```python
from build123d import *

# Parameters (mm, degrees)
F0_W     = 50.8
F0_H     = 38.1
F0_R     = 6.35
F1_DEPTH = 12.446
F2_W     = 1.417765
F2_H     = 38.1
F3_DEPTH = 2.54
F5_DEPTH = 38.1
F6_R     = 2.931554
F7_DEPTH = 12.7


with BuildPart() as f1:
    # F0 (on Top) → F1 (new body)
    with BuildSketch(Plane.XY):
        Rectangle(F0_W, F0_H)
        Circle(F0_R, mode=Mode.SUBTRACT)
    extrude(amount=F1_DEPTH)

    # F2 (on face) → F3 (cut)
    with BuildSketch(Plane.XY.offset(12.446)):
        with Locations((-17.610003, 0)):
            Rectangle(F2_W, F2_H)
        with BuildLine():
            Line((3.892783, 19.05), (0, 19.05))
            Line((0, 19.05), (0, 6.35))
            ThreePointArc((0, 6.35), (2.057368, 6.007473), (3.892783, 5.016846))
            Line((3.892783, 5.016846), (3.892783, 19.05))
        make_face()
        with BuildLine():
            Line((0, -6.35), (0, -19.05))
            Line((0, -19.05), (3.892783, -19.05))
            Line((3.892783, -19.05), (3.892783, -5.016846))
            ThreePointArc((3.892783, -5.016846), (2.057368, -6.007473), (0, -6.35))
        make_face()
    extrude(amount=-F3_DEPTH, mode=Mode.SUBTRACT)

    # F4 (on face) → F5 (cut)
    with BuildSketch(Plane.XZ.offset(19.05)):
        Polygon((14.809987, 12.446), (10.999987, 12.446), (8.067048, 7.366), (14.809987, 7.366), align=None)
        Polygon((18.619987, 12.446), (14.809987, 12.446), (14.809987, 7.366), (21.552927, 7.366), align=None)
    extrude(amount=-F5_DEPTH, mode=Mode.SUBTRACT)

    # F6 (on face) → F7 (join)
    with BuildSketch(Plane.YZ.offset(25.4)):
        with Locations((0, 6.223)):
            Circle(F6_R)
    extrude(amount=F7_DEPTH)


solid = f1.part
```
Geometry check sheet. Reference: the model listing, model coordinates, mm. A direction names the side the tool comes from. Round coordinates to 2 decimals unless told otherwise and drop trailing zeros. Order: outer loops, then holes, each group sorted by start corner. A loop starts at its lowest first (then second) coordinate and runs counter-clockwise, first axis right, second up. Notation, with made-up numbers: (9, 80.5) -> (58, 80.5) arc R33 ccw to (58, 118.5) -> close; hole circle Ø9 at (41.5, 8.5). An arc over 180 degrees is marked (long way). Return JSON: item names as keys, results as strings. Group by question number.
Q1. Section check D-D, the plane z = 5.5. Record the boundary of the cut face in (x, y), plus the area to 3 significant figures.
Q2. Section check C-C, the plane y = -7. Record the boundary of the cut face in (x, z), plus the area to 3 significant figures.
Q3. Section check A-A, the plane y = 0. Record the boundary of the cut face in (x, z), plus the area to 3 significant figures.
Q4. Tool access check on faces 1 (the flat face through (0, -13, 11)), 2 (the flat face through (15, 0, 7.366)), 3 (the flat face through (0, -19.05, 6)), 4 (the cylindrical face through (31.661, -0.636, 3.361)), 5 (the cylindrical face through (-6.344, 0.279, 6.136)). Record the directions out of +Z, -Z, +X, -X, +Y, -Y that give a thin tool (end or side, any length) a straight path to the whole face; none if there is none.
Q5. Gauge pin test, flat ends, axial feed: pin 1 (0.8 mm diameter, centred on y = 10, z = 11.5, fed in from +X); pin 2 (1.1 mm diameter, centred on x = -17.5, y = 1.5, fed in from +Z). Record the tip position at first contact, or that the pin passes through.
Q6. Release check for a two-part mould opening along X. For faces 6 (the flat face through (-18.319, 0, 11)), 7 (the flat face through (5, 5, 0)), 8 (the flat face through (25.4, 0, 2)) record: released by +X, released by -X, zero draft, split by the parting line, or undercut.
Q7. Section check B-B, the plane z = 11.5. Record the boundary of the cut face in (x, y).
Q8. Material ranges on probe 1 along Y at (x, z) = (0, 2.75); probe 2 along X at (y, z) = (0, 3.5); probe 3 along X at (y, z) = (10.5, 12.25), recorded low to high. Write a range as from..to.
Numbers:
{
 "1": {"outline": "(-25.4, -19.05) -> (25.4, -19.05) -> (25.4, -2.84) -> (38.1, -2.84) -> (38.1, 2.84) -> (25.4, 2.84) -> (25.4, 19.05) -> (-25.4, 19.05) -> close; hole circle Ø12.7 at (0, 0)", "area": "1,880 mm^2"},
 "2": {"outline": "(-25.4, 0) -> (25.4, 0) -> (25.4, 12.45) -> (18.62, 12.45) -> (21.55, 7.37) -> (8.07, 7.37) -> (11, 12.45) -> (3.89, 12.45) -> (3.89, 9.91) -> (0, 9.91) -> (0, 12.45) -> (-16.9, 12.45) -> (-16.9, 9.91) -> (-18.32, 9.91) -> (-18.32, 12.45) -> (-25.4, 12.45) -> close", "area": "565 mm^2"},
 "3": {"outline": "(-25.4, 0) -> (-6.35, 0) -> (-6.35, 12.45) -> (-16.9, 12.45) -> (-16.9, 9.91) -> (-18.32, 9.91) -> (-18.32, 12.45) -> (-25.4, 12.45) -> close; (6.35, 0) -> (25.4, 0) -> (25.4, 3.29) -> (38.1, 3.29) -> (38.1, 9.15) -> (25.4, 9.15) -> (25.4, 12.45) -> (18.62, 12.45) -> (21.55, 7.37) -> (8.07, 7.37) -> (11, 12.45) -> (6.35, 12.45) -> close", "area": "491 mm^2"},
 "4": {"face 1": "+Z, +Y, -Y", "face 2": "+Y, -Y", "face 3": "+Z, -Z, +X, -X, -Y", "face 4": "+X", "face 5": "+Z, -Z"},
 "5": {"pin 1": "x = 25.4", "pin 2": "z = 9.91"},
 "6": {"face 6": "undercut", "face 7": "zero draft", "face 8": "released by +X"},
 "7": {"outline": "(-25.4, -19.05) -> (-18.32, -19.05) -> (-18.32, 19.05) -> (-25.4, 19.05) -> close; (-16.9, -19.05) -> (0, -19.05) -> (0, -6.35) arc R6.35 cw to (0, 6.35) -> (0, 19.05) -> (-16.9, 19.05) -> close; (3.89, -19.05) -> (10.45, -19.05) -> (10.45, 19.05) -> (3.89, 19.05) -> (3.89, 5.02) arc R6.35 cw to (3.89, -5.02) -> close; (19.17, -19.05) -> (25.4, -19.05) -> (25.4, 19.05) -> (19.17, 19.05) -> close"},
 "8": {"probe 1": "-19.05..-6.35, 6.35..19.05", "probe 2": "-25.4..-6.35, 6.35..38.1", "probe 3": "-25.4..-18.32, -16.9..0, 3.89..10.89, 18.73..25.4"}
}
